Could you check a few things on this drawing? It's one solid part, dimensions in mm from its lowest x, y, z. A direction names the side the tool comes from. Give positions to 0.01 mm unless a question says otherwise; leave off trailing zeros. Order: outer loops, then holes, each group sorted by start corner. A loop starts at its lowest first (then second) coordinate and runs counter-clockwise, first axis right, second up.
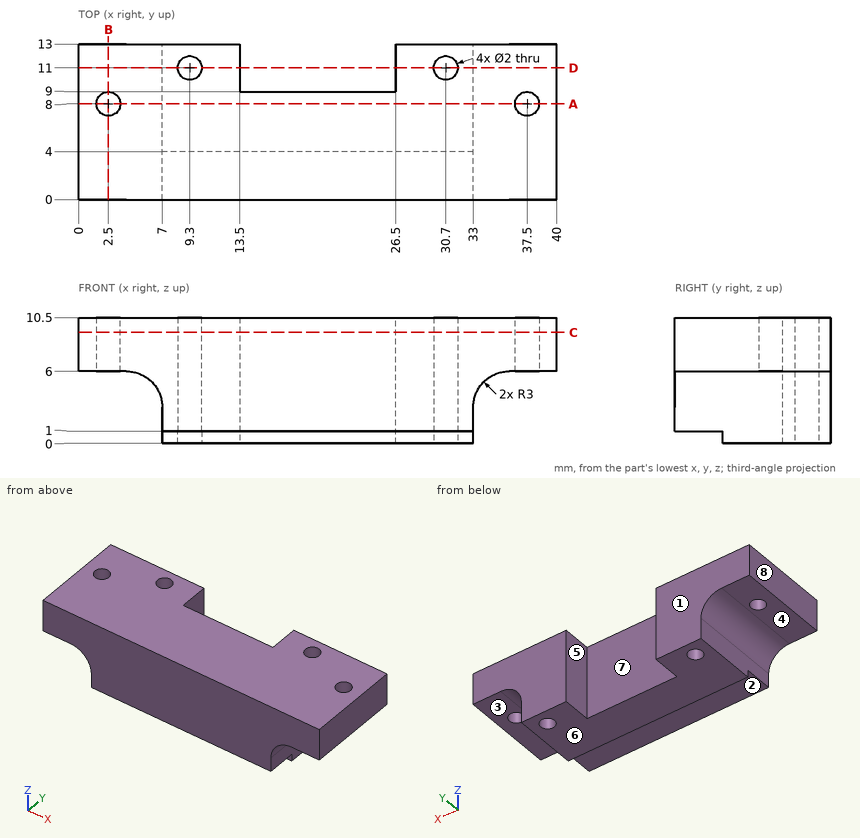
Q1. If we section it at A-A on y = 8: List the corners of the cut face in (x, z) for me.
Filled sheet:
outline: (0, 6) - (1.5, 6) - (1.5, 10.5) - (0, 10.5) - close; (3.5, 6) - (4, 6) arc R3 cw to (7, 3) - (7, 0) - (33, 0) - (33, 3) arc R3 cw to (36, 6) - (36.5, 6) - (36.5, 10.5) - (3.5, 10.5) - close; (38.5, 6) - (40, 6) - (40, 10.5) - (38.5, 10.5) - close
Q2. For the marked faces 1, 2, 3, 4 and 5, which set-ups out of +Z, -Z, +X, -X, +Y, -Y let a thin tool reach every point of the face, with its end or its side?
Filled sheet:
face 1: +Z, -Z, +X, -X, +Y
face 2: -Z, +X, -X, -Y
face 3: -Z, +X, +Y, -Y
face 4: -Z, -X, +Y, -Y
face 5: +Z, -Z, +Y
Q3. If we section it at B-B on x = 2.5: List the corners of the cut face in (y, z) for me, plus the area to 3 significant figures.
Filled sheet:
outline: (0, 6) - (7, 6) - (7, 10.5) - (0, 10.5) - close; (9, 6) - (13, 6) - (13, 10.5) - (9, 10.5) - close
area: 49.5 mm2
Q4. Thinking about a two-plate mould opening in X: for the marked faces 6, 7 and 8, which applies, released by +X, released by -X, zero draft, split by the parting line, or undercut?
Filled sheet:
face 6: zero draft
face 7: undercut
face 8: released by -X
Q5. I need wall thicknesses on L1, parallel to Y at x = 2.5, z = 8.3; L2, parallel to Y at x = 30.7, z = 5.75; L3, parallel to Z at x = 14, y = 3.5. Which ranges of each line are inside material? Lowest first, please.
Filled sheet:
L1: y = 0 to 7, 9 to 13
L2: y = 0 to 10, 12 to 13
L3: z = 1 to 10.5
Q6. I'm going to push flat-ended pins straight in: P1, Ø4.5, axis at x = 38.5, y = 4, coming from the -Z side; P2, Ø0.5, axis at x = 15, z = 0.5, coming from the -Y side; P3, Ø1.2, axis at x = 25.5, y = 2, coming from the -Z side. Where does each tip first touch, or does it pass through?
Filled sheet:
P1: stops at z = 6
P2: stops at y = 4
P3: stops at z = 1
Q7. If we section it at D-D on y = 11: List the corners of the cut face in (x, z) for me, plus the area to 3 significant figures.
Filled sheet:
outline: (0, 6) - (4, 6) arc R3 cw to (7, 3) - (7, 0) - (8.3, 0) - (8.3, 10.5) - (0, 10.5) - close; (10.3, 0) - (13.5, 0) - (13.5, 10.5) - (10.3, 10.5) - close; (26.5, 0) - (29.7, 0) - (29.7, 10.5) - (26.5, 10.5) - close; (31.7, 0) - (33, 0) - (33, 3) arc R3 cw to (36, 6) - (40, 6) - (40, 10.5) - (31.7, 10.5) - close
area: 161 mm2
Q8. If we section it at C-C on z = 9.25: List the corners of the cut face in (x, y) for me, plus the area to 3 significant figures.
Filled sheet:
outline: (0, 0) - (40, 0) - (40, 13) - (26.5, 13) - (26.5, 9) - (13.5, 9) - (13.5, 13) - (0, 13) - close; hole circle Ø2 at (2.5, 8); hole circle Ø2 at (9.3, 11); hole circle Ø2 at (30.7, 11); hole circle Ø2 at (37.5, 8)
area: 455 mm2
